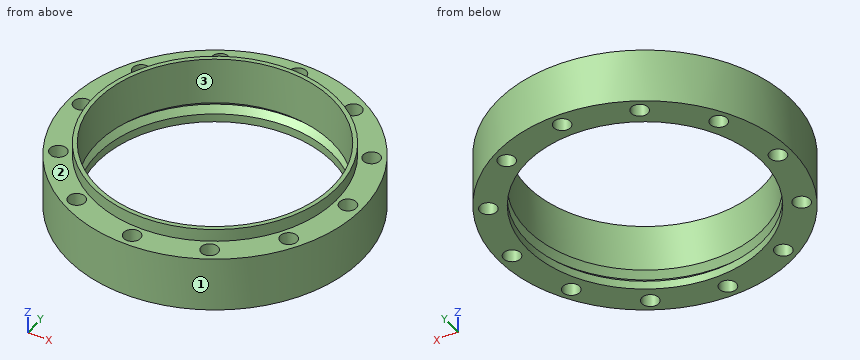
from build123d import *

# Parameters (mm, degrees)
SKETCH_1_R               = 35
EXTRUDE_1_DEPTH          = 16
SKETCH_2_R               = 35
SKETCH_2_R_2             = 29
CUT_EXTRUDE_1_DEPTH      = 3
SKETCH_3_R               = 28
CUT_EXTRUDE_2_DEPTH      = 17
SKETCH_4_R               = 2
CUT_EXTRUDE_3_DEPTH      = 14
PATTERN_CIRCULAR_1_COUNT = 12


with BuildPart() as part:
    # 草图1 → 凸台-拉伸1 (new body)
    with BuildSketch(Plane.XY):
        Circle(SKETCH_1_R)
    extrude(amount=EXTRUDE_1_DEPTH)

    # 草图2 → 切除-拉伸1 (cut)
    with BuildSketch(Plane.XY.offset(16)):
        Circle(SKETCH_2_R)
        Circle(SKETCH_2_R_2, mode=Mode.SUBTRACT)
    extrude(amount=-CUT_EXTRUDE_1_DEPTH, mode=Mode.SUBTRACT)

    # 草图3 → 切除-拉伸2 (cut, through all)
    with BuildSketch(Plane.XY.offset(16)):
        Circle(SKETCH_3_R)
    extrude(amount=-CUT_EXTRUDE_2_DEPTH, mode=Mode.SUBTRACT)

    # 草图4 → 切除-拉伸3 (cut, through all)
    with BuildSketch(Plane.XY.offset(13)):
        with Locations((0, 31.847890671)):
            Circle(SKETCH_4_R)
    cut_extrude_3 = extrude(amount=-CUT_EXTRUDE_3_DEPTH, mode=Mode.SUBTRACT)

    # 阵列(圆周)1: 切除-拉伸3 ×12 about axis
    pattern_circular_1_axis = Axis((0, 0, 0), (0, 0, 1))
    for i in range(1, PATTERN_CIRCULAR_1_COUNT):
        add(cut_extrude_3.rotate(pattern_circular_1_axis, i * 360 / PATTERN_CIRCULAR_1_COUNT), mode=Mode.SUBTRACT)

    # 草图5 → 切除-旋转3 (revolve, cut)
    with BuildSketch(Plane(origin=(0, 0, 0), x_dir=(0, 0, -1), z_dir=(1, 0, 0))):
        Polygon((-4.855352657, 27.98817223), (-1.98280478, 27.986477885), (-3.419925891, 29.423598996), align=None)
    revolve(axis=Axis((0, 0, 0), (0, 0, 1)), mode=Mode.SUBTRACT)


solid = part.part
CAD build for the part. Positions are in the model's coordinates, mm. Face numbers are marked on the shaded views. Round coordinates to 2 decimals unless told otherwise and drop trailing zeros. Order: outer loops, then holes, each group sorted by start corner. A loop starts at its lowest first (then second) coordinate and runs counter-clockwise, first axis right, second up. Notation, with made-up numbers: (2.5, 83.25) - (8.5, 83.25) arc R11 ccw to (8.5, 94.25) - close; hole circle Ø6 at (67, 48). An arc over 180 degrees is marked (long way). Return JSON: item names as keys, results as strings.
(1) Pin check, flat tips, straight feed: pin 1 Ø5 at (x, y) = (27.58, -15.92) entering from +Z; pin 2 Ø3.5 at (x, y) = (-15.92, -27.58) entering from -Z; pin 3 Ø1 at (y, z) = (9, 8.5) entering from +X; pin 4 Ø5 at (y, z) = (-11.5, 6.5) entering from -X. Stop position of each tip, or through.
Answer key:
{"pin 1": "stops at z = 13", "pin 2": "passes through", "pin 3": "stops at x = 33.95", "pin 4": "stops at x = -33.82"}
(2) Cut at C-C (z = 14.75). Give the cut face in (x, y), then the cut area to 3 significant figures.
Answer key:
{"outline": "circle Ø58 at (0, 0); hole circle Ø56 at (0, 0)", "area": "179 mm^2"}
(3) Pull direction Y, two halves, no side cores. Call the marked faces 1, 2 and 3: +Y half, -Y half, draft (parallel to the pull), parting line (faces both ways), or undercut.
Answer key:
{"face 1": "parting line", "face 2": "draft", "face 3": "undercut"}
(4) Wall check: probe 1 along Y at (x, z) = (0, 1.25); probe 2 along X at (y, z) = (29, 1.5); probe 3 along Z at (x, y) = (-21, 26.5). Give the ranges that are in metal, low to high. Write a range as from..to.
Answer key:
{"probe 1": "y = -35..-33.85, -29.85..-28, 28..29.85, 33.85..35", "probe 2": "x = -19.6..-17.33, -14.51..14.51, 17.33..19.6", "probe 3": "z = 0..13"}
(5) Cut at A-A (x = 0). Give the cut face in (y, z).
Answer key:
{"outline": "(-35, 0) - (-33.85, 0) - (-33.85, 13) - (-35, 13) - close; (-29.85, 0) - (-28, 0) - (-28, 2) - (-29.42, 3.42) - (-28, 4.84) - (-28, 16) - (-29, 16) - (-29, 13) - (-29.85, 13) - close; (28, 0) - (29.85, 0) - (29.85, 13) - (29, 13) - (29, 16) - (28, 16) - (28, 4.84) - (29.42, 3.42) - (28, 2) - close; (33.85, 0) - (35, 0) - (35, 13) - (33.85, 13) - close"}
(6) Cut at D-D (z = 8.75). State how many separate pieces and enclosed holes the cut face has, then the cut area to 3 significant figures.
Answer key:
{"separate pieces": "1", "enclosed holes": "13", "area": "1,230 mm^2"}
